Answer from the drawing. Dimensions are ordinates in mm from the lowest x, y and z of the part. Give positions to 0.01 mm unless a question says otherwise; leave off trailing zeros. Loops run counter-clockwise (first coordinate to the right, second up) from the corner with the lowest first, then second, coordinate; pieces in that order, holes last. Notation, with made-up numbers: (22.25, 59) - (54.25, 59) arc R33 cw to (54.25, 96) - close; hole circle Ø2 at (-2.75, 33.5). An arc over 180 degrees is marked (long way). Put each result on its own line as item: value. Start each with the question number.
1. Consider L1, parallel to Z at x = 12.5, y = 3.55; L2, parallel to Y at x = 2.5, z = 16; L3, parallel to Y at x = 9.5, z = 3. Determine where each line is inside the solid, lowest interval first. Write a range as from..to.
2. A cutting plane is placed at B-B, the plane y = 4.5. Determine the outline of the cut face in (x, z).
3. A cutting plane is placed at D-D, the plane y = 7.25. Determine the outline of the cut face in (x, z).
4. For a pull along Z with two mould halves and no side action, classify the marked faces 1, 2 and 3 as released by +Z, released by -Z, zero draft, split by the parting line, or undercut.
5. A cutting plane is placed at C-C, the plane z = 12.5. Determine the outline of the cut face in (x, y), plus the area to 3 significant figures.
6. Given pin 1 Ø1.5 at (x, y) = (10, 8) entering from -Z; pin 2 Ø5 at (x, y) = (21, 6.5) entering from +Z; pin 3 Ø6 at (x, y) = (13.5, 1) entering from -Z; pin 4 Ø2 at (x, y) = (20.5, 8.5) entering from +Z, each flat-ended and moving along its own axis, determine where each tip first touches the part or whether it passes through.
7. A cutting plane is placed at A-A, the plane x = 12.5. Determine the outline of the cut face in (y, z), plus the area to 3 significant figures.
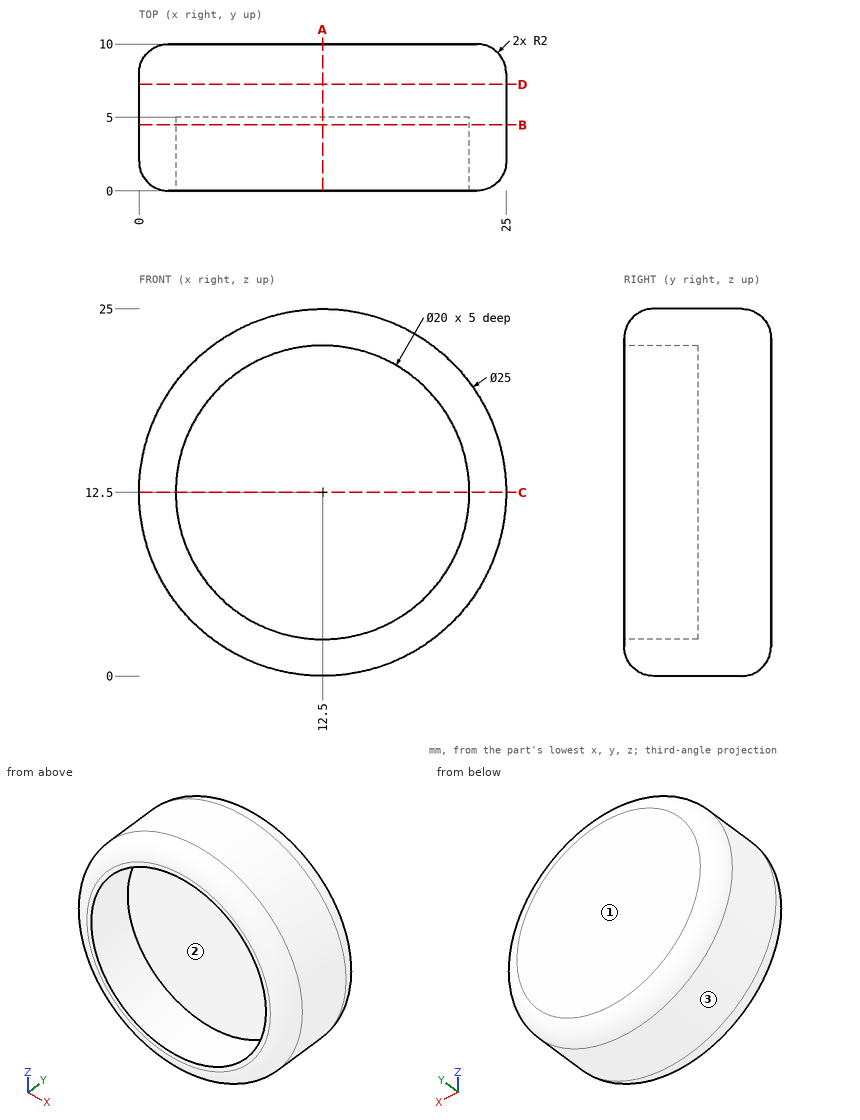
Return value:
1. L1: z = 0..2.5, 22.5..25
1. L2: y = 0..10
1. L3: y = 5..10
2. outline: circle Ø25 at (12.5, 12.5); hole circle Ø20 at (12.5, 12.5)
3. outline: circle Ø25 at (12.5, 12.5)
4. face 1: zero draft
4. face 2: undercut
4. face 3: split by the parting line
5. outline: (0, 2) arc R2 ccw to (2, 0) - (2.5, 0) - (2.5, 5) - (22.5, 5) - (22.5, 0) - (23, 0) arc R2 ccw to (25, 2) - (25, 8) arc R2 ccw to (23, 10) - (2, 10) arc R2 ccw to (0, 8) - close
5. area: 147 mm2
6. pin 1: stops at z = 0.12
6. pin 2: stops at z = 23.47
6. pin 3: stops at z = 0
6. pin 4: stops at z = 22.82
7. outline: (0, 2) arc R2 ccw to (2, 0) - (8, 0) arc R2 ccw to (10, 2) - (10, 23) arc R2 ccw to (8, 25) - (2, 25) arc R2 ccw to (0, 23) - (0, 22.5) - (5, 22.5) - (5, 2.5) - (0, 2.5) - close
7. area: 147 mm2
